Can you work these out from the model? Positions are in its coordinate system, mm. Face numbers are marked on the shaded views. A direction names the side the tool comes from. Give positions to 0.01 mm unless a question says otherwise; leave off trailing zeros. Order: outer loops, then holes, each group sorted by start corner. A loop starts at its lowest first (then second) coordinate and runs counter-clockwise, first axis right, second up. Notation, with made-up numbers: (-36, 19.25) -> (-30, 19.25) arc R14 cw to (-30, 33.25) -> close; hole circle Ø2 at (53, -9). An arc over 180 degrees is marked (long way). Answer as CSV lines item,"result".
```python
from build123d import *

# Parameters (mm, degrees)
F0_W          = 50.8
F0_H          = 50.8
F1_DEPTH      = 2.54
F1_DEPTH_BACK = 2.54
F2_W          = 40.64
F2_H          = 40.64
F3_DEPTH      = 5.081
F4_W          = 50.8
F4_H          = 50.8
F5_DEPTH      = 2.54
F5_DEPTH_BACK = 2.54


with BuildPart() as f1:
    # F0 (on Top) → F1 (new body, two sides)
    with BuildSketch(Plane.XY) as f1_sk:
        Rectangle(F0_W, F0_H)
    extrude(amount=F1_DEPTH)
    extrude(f1_sk.sketch, amount=-F1_DEPTH_BACK)

    # F2 (on face) → F3 (cut, through all)
    with BuildSketch(Plane.XY.offset(2.54)):
        Rectangle(F2_W, F2_H)
    extrude(amount=-F3_DEPTH, mode=Mode.SUBTRACT)

    # F4 (on Front) → F5 (join, two sides)
    with BuildSketch(Plane.XZ) as f5_sk:
        Rectangle(F4_W, F4_H)
    extrude(amount=F5_DEPTH)
    extrude(f5_sk.sketch, amount=-F5_DEPTH_BACK)


solid = f1.part
```
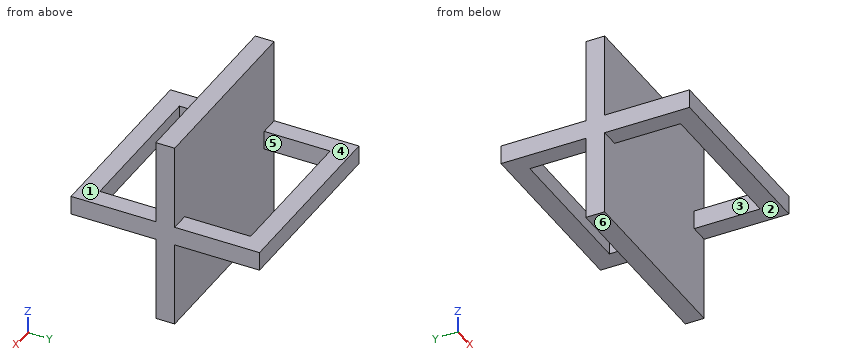
Item 1: For pin 1 (6 mm diameter, centred on x = 9.5, z = 7, fed in from +Y); pin 2 (18.5 mm diameter, centred on x = -7, y = -14, fed in from -Z); pin 3 (6 mm diameter, centred on x = 19.5, z = 7.5, fed in from -Y), each with a flat end and sliding along its axis, tell me the tip position at first contact or that it passes through.
Numbers:
pin 1,"stops at y = 2.54"
pin 2,"stops at z = -2.54"
pin 3,"stops at y = -2.54"
Item 2: For the marked faces 1, 2, 3 and 4, which set-ups out of +Z, -Z, +X, -X, +Y, -Y let a thin tool reach every point of the face, with its end or its side?
Numbers:
face 1,"+Z, +X, -X, -Y"
face 2,"-Z, +X, -X, -Y"
face 3,"+Z, -Z"
face 4,"+Z, +X, -X, +Y"
Item 3: Imagine slicing it at C-C, the plane x = -21.5. Please give me the cut outline in (y, z), then the cut area to 3 significant figures.
Numbers:
outline,"(-25.4, -2.54) -> (-2.54, -2.54) -> (-2.54, -25.4) -> (2.54, -25.4) -> (2.54, -2.54) -> (25.4, -2.54) -> (25.4, 2.54) -> (2.54, 2.54) -> (2.54, 25.4) -> (-2.54, 25.4) -> (-2.54, 2.54) -> (-25.4, 2.54) -> close"
area,"490 mm²"
Item 4: Imagine slicing it at D-D, the plane z = 13.5. Please give me the cut outline in (x, y).
Numbers:
outline,"(-25.4, -2.54) -> (25.4, -2.54) -> (25.4, 2.54) -> (-25.4, 2.54) -> close"
Item 5: Imagine slicing it at A-A, the plane x = 9.5. Please give me the cut outline in (y, z), then the cut area to 3 significant figures.
Numbers:
outline,"(-25.4, -2.54) -> (-20.32, -2.54) -> (-20.32, 2.54) -> (-25.4, 2.54) -> close; (-2.54, -25.4) -> (2.54, -25.4) -> (2.54, 25.4) -> (-2.54, 25.4) -> close; (20.32, -2.54) -> (25.4, -2.54) -> (25.4, 2.54) -> (20.32, 2.54) -> close"
area,"310 mm²"
Item 6: We'd pull the mould along Y, two halves only. Please class the marked faces 5 and 6: released by +Y, released by -Y, zero draft, split by the parting line, or undercut.
Numbers:
face 5,"undercut"
face 6,"zero draft"
Item 7: Please list where this line runs through material, in increasing order: line 1 along Y through (x, z) = (-18.5, 23).
Numbers:
line 1,"y = -2.54 to 2.54"
Item 8: Imagine slicing it at B-B, the plane y = 13. Please give me the cut outline in (x, z).
Numbers:
outline,"(-25.4, -2.54) -> (-20.32, -2.54) -> (-20.32, 2.54) -> (-25.4, 2.54) -> close; (20.32, -2.54) -> (25.4, -2.54) -> (25.4, 2.54) -> (20.32, 2.54) -> close"
